Work out the finished part from the listing and answer in its coordinate system (mm). Face numbers are marked on the shaded views. A direction names the side the tool comes from. Coordinates: 2 decimals unless noted, no trailing zeros. Order: outer loops, then holes, each group sorted by start corner. A loop starts at its lowest first (then second) coordinate and runs counter-clockwise, first axis right, second up. Notation, with made-up numbers: (-6.75, 46) -> (34.25, 46) arc R15 ccw to (34.25, 69) -> close; hole circle Ø11 at (-35, -14). An arc over 180 degrees is marked (long way). Write item = value, one per line. Start each with the question number.
Q1. Which of the six approach directions +Z, -Z, +X, -X, +Y, -Y give full straight-line access (tool end or side, diameter ignored) to the marked faces 4, 5, 6, 7 and 8?
Q2. Flat-ended cylindrical pins translate along their axes: pin 1 (4 mm diameter, centred on y = 7.5, z = -17.5, fed in from -X); pin 2 (1 mm diameter, centred on x = 3, z = -10, fed in from -Y); pin 3 (3 mm diameter, centred on x = 2.5, z = -18.5, fed in from +Y). Find the tip coordinate at first contact, or state that the pin passes through.
Q3. The part is cut by section C-C, the plane z = -4. Determine the outline of the cut face in (x, y).
Q4. The part is cut by section B-B, the plane y = 7.5. Determine the outline of the cut face in (x, z).
Q5. For a pull along Y with two mould halves and no side action, classify the marked faces 1, 2 and 3 as +Y half, -Y half, draft (parallel to the pull), parting line (faces both ways), or undercut.
Q6. The part is cut by section D-D, the plane y = 4.75. Determine the outline of the cut face in (x, z).
Q7. The part is cut by section A-A, the plane x = 2.75. Determine the outline of the cut face in (y, z).
Q8. Straight lines are drawn through the part: L1, parallel to Y at x = 6.5, z = -13.25; L2, parallel to Z at x = 7.5, y = 7.5. For each, find the intervals that lie inside material, in ascending order. Write a range as from..to.
Autodesk Fusion 360 part; units mm, degrees
sketch "Sketch1" plane through (0, 0, 0) normal (0, 0, 1) x (1, 0, 0)
  line L0 (0, 0) -> (8.5, 0)
  line L1 (8.5, 0) -> (8.5, 8.5)
  line L2 (8.5, 8.5) -> (0, 8.5)
  line L3 (0, 8.5) -> (0, 0)
  dimension "d1" = 8.5
extrude "Extrude1" add sketch "Sketch1" along normal blind 3
sketch "Sketch2" plane through (0, 0, 0) normal (0, 0, -1) x (1, 0, 0)
  line L0 (0, 0) -> (0, -8.5)
  line L1 (0, -8.5) -> (8.5, -8.5)
  line L2 (8.5, -8.5) -> (8.5, 0)
  line L3 (8.5, 0) -> (0, 0)
  line L4 (0.5, -0.5) -> (8, -0.5)
  line L5 (8, -0.5) -> (8, -8)
  line L6 (8, -8) -> (0.5, -8)
  line L7 (0.5, -8) -> (0.5, -0.5)
  line L8 (0.5, -0.5) -> (8, -8) construction
  line L9 (8.5, 0) -> (0, -8.5) construction
  dimension "d4" = 7.5
extrude "Extrude2" add sketch "Sketch2" along normal blind 23 contours L4 L5 L6 L7
sketch "Sketch3" plane through (8, 0, 0) normal (1, 0, 0) x (0, 1, 0)
  line L0 (8, 0) -> (0.5, 0)
  line L1 (0.5, 0) -> (0.5, -23)
  line L2 (0.5, -23) -> (8, -23)
  line L3 (8, -23) -> (8, 0)
  line L4 (0.5, -23) -> (4.25, -20.8349)
  line L5 (4.25, -20.8349) -> (8, -23)
  line L6 (8, -23) -> (0.5, -23)
  dimension "d7" = 120
extrude "Extrude3" cut sketch "Sketch3" against normal through all contours L2 L4 L5 L6
fillet "Fillet1" radius 1 2 edges at (4.25, 0.5, -23) (4.25, 8, -23)
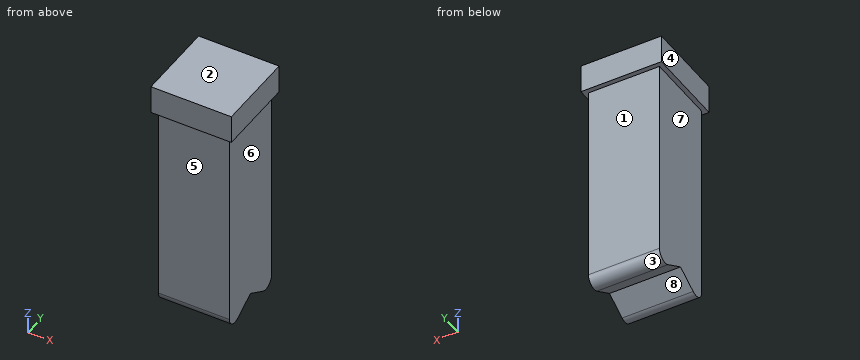
Model answer:
q1.face_4 = +Z, -Z, -X, +Y, -Y
q1.face_5 = -Z, +X, -X, -Y
q1.face_6 = -Z, +X, +Y, -Y
q1.face_7 = -Z, -X, +Y, -Y
q1.face_8 = -Z, +X, -X
q2.pin_1 = 0.5
q2.pin_2 = 0.5
q2.pin_3 = 8
q3.outline = (0.5, 0.5) -> (8, 0.5) -> (8, 8) -> (0.5, 8) -> close
q4.outline = (0, 0) -> (0.5, 0) -> (0.5, -22.13) -> (8, -22.13) -> (8, 0) -> (8.5, 0) -> (8.5, 3) -> (0, 3) -> close
q5.face_1 = +Y half
q5.face_2 = draft
q5.face_3 = undercut
q6.outline = (0, 0) -> (0.5, 0) -> (0.5, -21.12) -> (8, -21.12) -> (8, 0) -> (8.5, 0) -> (8.5, 3) -> (0, 3) -> close
q7.outline = (0, 0) -> (0.5, 0) -> (0.5, -21.27) arc R1 ccw to (2, -22.13) -> (4.25, -20.83) -> (6.5, -22.13) arc R1 ccw to (8, -21.27) -> (8, 0) -> (8.5, 0) -> (8.5, 3) -> (0, 3) -> close
q8.L1 = 0.5..8
q8.L2 = -22.13..3
